from build123d import *

# Parameters (mm, degrees)
SKETCH2_R           = 3.1
SKETCH2_R_2         = 1.7
BOSS_EXTRUDE1_DEPTH = 5
FILLET1_R           = 10
FILLET2_R           = 2
SKETCH3_W           = 10
SKETCH3_H           = 40
CUT_EXTRUDE1_DEPTH  = 5
FILLET3_R           = 4


with BuildPart() as part:
    # Sketch2 → Boss-Extrude1 (new body)
    with BuildSketch(Plane.YZ):
        Polygon((-20, 0), (-20, 94), (-34, 94), (-34, 114), (34, 114), (34, 94), (20, 94), (20, 0), align=None)
        with Locations(Location((0, 40, 0), (0, 0, 270))):
            Circle(SKETCH2_R, mode=Mode.SUBTRACT)
        with Locations(Location((-24, 104, 0), (0, 0, 270))):
            Circle(SKETCH2_R_2, mode=Mode.SUBTRACT)
        with Locations(Location((24, 104, 0), (0, 0, 270))):
            Circle(SKETCH2_R_2, mode=Mode.SUBTRACT)
    extrude(amount=BOSS_EXTRUDE1_DEPTH)

    # Fillet1
    fillet1_edges = [part.edges().sort_by_distance(p)[0] for p in [
        (2.5, -20, 94),
        (2.5, 20, 94),
    ]]
    fillet(fillet1_edges, radius=FILLET1_R)

    # Fillet2
    fillet2_edges = [part.edges().sort_by_distance(p)[0] for p in [
        (2.5, -34, 94),
        (2.5, -34, 114),
        (2.5, 34, 114),
        (2.5, 34, 94),
    ]]
    fillet(fillet2_edges, radius=FILLET2_R)

    # Sketch3 → Cut-Extrude1 (cut)
    with BuildSketch(Plane(origin=(0, 0, 0), x_dir=(0, -1, 0), z_dir=(-1, 0, 0))):
        with Locations((0, 94)):
            Rectangle(SKETCH3_W, SKETCH3_H)
    extrude(amount=-CUT_EXTRUDE1_DEPTH, mode=Mode.SUBTRACT)

    # Fillet3
    fillet3_edges = [part.edges().sort_by_distance(p)[0] for p in [
        (2.5, 5, 74),
        (2.5, 5, 114),
        (2.5, -5, 114),
        (2.5, -5, 74),
    ]]
    fillet(fillet3_edges, radius=FILLET3_R)


solid = part.part
Build history of the part. All positions in model axes, mm. A direction names the side the tool comes from. Give positions to 0.01 mm unless a question says otherwise; leave off trailing zeros. Loops run counter-clockwise (first coordinate to the right, second up) from the corner with the lowest first, then second, coordinate; pieces in that order, holes last. Notation, with made-up numbers: (-13.5, -11.5) -> (20.5, -11.5) arc R23 ccw to (20.5, -0.5) -> close; hole circle Ø5 at (-5, -8). An arc over 180 degrees is marked (long way). Answer in a Markdown table with one row per item.
Item 1: Slice it at A-A on x = 3.9. Write the cut outline in (y, z), plus the area to 3 significant figures.
Findings below:
| item | result |
|---|---|
| outline | (-34, 96) arc R2 ccw to (-32, 94) -> (-30, 94) arc R10 cw to (-20, 84) -> (-20, 0) -> (20, 0) -> (20, 84) arc R10 cw to (30, 94) -> (32, 94) arc R2 ccw to (34, 96) -> (34, 112) arc R2 ccw to (32, 114) -> (9, 114) arc R4 ccw to (5, 110) -> (5, 78) arc R4 cw to (1, 74) -> (-1, 74) arc R4 cw to (-5, 78) -> (-5, 110) arc R4 ccw to (-9, 114) -> (-32, 114) arc R2 ccw to (-34, 112) -> close; hole circle Ø3.4 at (-24, 104); hole circle Ø6.2 at (0, 40); hole circle Ø3.4 at (24, 104) |
| area | 4,710 mm² |
Item 2: Tool access for faces 1 (the flat face through (2, -20, 41)), 2 (the flat face through (2, 34, 104)), 3 (the flat face through (2, 20, 43)), 4 (the flat face through (2, -5, 94)), 5 (the flat face through (5, 0, 58)): list every direction of +Z, -Z, +X, -X, +Y, -Y with a clear straight run to the whole face (end or side of a thin tool).
Findings below:
| item | result |
|---|---|
| face 1 | -Z, +X, -X, -Y |
| face 2 | +Z, -Z, +X, -X, +Y |
| face 3 | -Z, +X, -X, +Y |
| face 4 | +Z, +X, -X |
| face 5 | +Z, -Z, +X, +Y, -Y |
Item 3: Probe line 1 along Y through (x, z) = (3.95, 104); line 2 along Y through (x, z) = (2.4, 100.5); line 3 along Y through (x, z) = (2.05, 80). List the from-to ranges inside material, lowest first. Write a range as [from, to].
Findings below:
| item | result |
|---|---|
| line 1 | y = [-34, -25.7], [-22.3, -5], [5, 22.3], [25.7, 34] |
| line 2 | y = [-34, -5], [5, 34] |
| line 3 | y = [-20, -5], [5, 20] |
Item 4: Slice it at C-C on z = 104. Write the cut outline in (x, y).
Findings below:
| item | result |
|---|---|
| outline | (0, -34) -> (5, -34) -> (5, -25.7) -> (0, -25.7) -> close; (0, -22.3) -> (5, -22.3) -> (5, -5) -> (0, -5) -> close; (0, 5) -> (5, 5) -> (5, 22.3) -> (0, 22.3) -> close; (0, 25.7) -> (5, 25.7) -> (5, 34) -> (0, 34) -> close |
Item 5: Flat gauge pins, fed straight in: P1, Ø2, axis at x = 1, y = 3.5, coming from the +Z side; P2, Ø3, axis at x = 0.5, z = 20.5, coming from the +Y side; P3, Ø1.6, axis at x = 2, y = -0.5, coming from the +Z side; P4, Ø5, axis at y = 0, z = 40, coming from the -X side. Where does each tip first touch, or does it go through?
Findings below:
| item | result |
|---|---|
| P1 | stops at z = 76.06 |
| P2 | stops at y = 20 |
| P3 | stops at z = 74.01 |
| P4 | passes through |
Item 6: Slice it at B-B on y = 24. Write the cut outline in (x, z), plus the area to 3 significant figures.
Findings below:
| item | result |
|---|---|
| outline | (0, 92) -> (5, 92) -> (5, 102.3) -> (0, 102.3) -> close; (0, 105.7) -> (5, 105.7) -> (5, 114) -> (0, 114) -> close |
| area | 93.0 mm² |
Item 7: Slice it at D-D on z = 68.5. Write the cut outline in (x, y).
Findings below:
| item | result |
|---|---|
| outline | (0, -20) -> (5, -20) -> (5, 20) -> (0, 20) -> close |
Item 8: Mould opens along Z. For faces 6 (the cylindrical face through (2.46, 24.07, 105.7)), 7 (the flat face through (2, 0, 74)), 8 (the cylindrical face through (2.54, 33.4, 94.57)) say: pulls with the +Z half, pulls with the -Z half, needs draft (parallel to the pull), parting line crosses it, or undercut.
Findings below:
| item | result |
|---|---|
| face 6 | undercut |
| face 7 | pulls with the +Z half |
| face 8 | pulls with the -Z half |
